For this review, take the finished solid that the model builds, in its own axes (mm). A direction names the side the tool comes from. Round coordinates to 2 decimals unless told otherwise and drop trailing zeros. Order: outer loops, then holes, each group sorted by start corner. A loop starts at its lowest first (then second) coordinate and runs counter-clockwise, first axis right, second up. Notation, with made-up numbers: M 1,62 L 12,62 A19 ccw 12,76 Z; hole C 73.5,-38.75 d3. An arc over 180 degrees is marked long. Use a Markdown table: item, result.
from build123d import *

# Parameters (mm, degrees)
SKETCH1_R           = 1.75
SKETCH1_W           = 3
SKETCH1_H           = 10
BOSS_EXTRUDE1_DEPTH = 3


with BuildPart() as part:
    # Sketch1 → Boss-Extrude1 (new body)
    with BuildSketch(Plane(origin=(0, 0, 0), x_dir=(1, 0, 0), z_dir=(0, 1, 0))):
        with BuildLine():
            Line((-32.051716829, -25), (-32.051716829, 2.5))
            ThreePointArc((-32.051716829, 2.5), (-34.980649017, 9.571067812), (-42.051716829, 12.5))
            Line((-42.051716829, 12.5), (-62.5, 12.5))
            ThreePointArc((-62.5, 12.5), (-64.267766953, 11.767766953), (-65, 10))
            Line((-65, 10), (-65, -10))
            ThreePointArc((-65, -10), (-64.267766953, -11.767766953), (-62.5, -12.5))
            Line((-62.5, -12.5), (-51.731989821, -12.5))
            ThreePointArc((-51.731989821, -12.5), (-47.304406502, -13.946364237), (-44.584529361, -17.727598413))
            Line((-44.584529361, -17.727598413), (-41.943571372, -26.034291608))
            ThreePointArc((-41.943571372, -26.034291608), (-36.531751789, -29.972890141), (-32.051716829, -25))
        make_face()
        with Locations(Location((-45, 0, 0), (0, 0, 270))):
            Circle(SKETCH1_R, mode=Mode.SUBTRACT)
        with Locations(Location((-37.051716829, -25, 0), (0, 0, 270))):
            Circle(SKETCH1_R, mode=Mode.SUBTRACT)
        with Locations((-59, 0)):
            Rectangle(SKETCH1_W, SKETCH1_H, mode=Mode.SUBTRACT)
    extrude(amount=BOSS_EXTRUDE1_DEPTH)


solid = part.part
Q1. Wall thickness on line 1 along X through (y, z) = (2.15, 0); line 2 along X through (y, z) = (1.75, 25); line 3 along Z through (x, y) = (-59, 0.7): over which ranges is each line inside the solid? List them lowest first. Write a range as [from, to].
Determined:
| item | result |
|---|---|
| line 1 | x = [-65, -60.5], [-57.5, -46.75], [-43.25, -32.05] |
| line 2 | x = [-42.27, -38.8], [-35.3, -32.05] |
| line 3 | z = [-12.5, -5], [5, 12.5] |
Q2. Add section C-C (x = -53.5). Write out the cut boundary in (y, z).
Determined:
| item | result |
|---|---|
| outline | M 0,-12.5 L 3,-12.5 L 3,12.5 L 0,12.5 Z |
Q3. Add section A-A (z = 0). Write out the cut boundary in (x, y).
Determined:
| item | result |
|---|---|
| outline | M -65,0 L -60.5,0 L -60.5,3 L -65,3 Z; M -57.5,0 L -46.75,0 L -46.75,3 L -57.5,3 Z; M -43.25,0 L -32.05,0 L -32.05,3 L -43.25,3 Z |
Q4. Add section B-B (y = 2.1). Write out the cut boundary in (x, z), then the cut area to 3 significant figures.
Determined:
| item | result |
|---|---|
| outline | M -65,-10 A2.5 ccw -62.5,-12.5 L -42.05,-12.5 A10 ccw -32.05,-2.5 L -32.05,25 A5 ccw -41.94,26.03 L -44.58,17.73 A7.5 cw -51.73,12.5 L -62.5,12.5 A2.5 ccw -65,10 Z; hole M -60.5,-5 L -57.5,-5 L -57.5,5 L -60.5,5 Z; hole C -45,0 d3.5; hole C -37.05,25 d3.5 |
| area | 948 mm^2 |
Q5. Draft analysis for pull direction X (two halves, no side actions). For faces 1 (the cylindrical face through (-64, 1, 12)), 2 (the flat face through (-45, 0, 4)), 3 (the cylindrical face through (-36.97, 1.48, 23.25)), 4 (the cylindrical face through (-37, 1, 30)), state which applies: pulls with the +X half, pulls with the -X half, needs draft (parallel to the pull), parting line crosses it, or undercut.
Determined:
| item | result |
|---|---|
| face 1 | pulls with the -X half |
| face 2 | needs draft |
| face 3 | undercut |
| face 4 | parting line crosses it |
Q6. Clearance check with flat-ended pins moving along their axes: pin 1 (1.5 mm diameter, centred on x = -59, y = 2, fed in from +Z); pin 2 (1 mm diameter, centred on x = -40.5, y = 0.5, fed in from -Z). State where each tip first meets the part, or that it passes through.
Determined:
| item | result |
|---|---|
| pin 1 | stops at z = 12.5 |
| pin 2 | stops at z = -12.44 |
Q7. Add section D-D (z = 13.5). Write out the cut boundary in (x, y).
Determined:
| item | result |
|---|---|
| outline | M -47.99,0 L -32.05,0 L -32.05,3 L -47.99,3 Z |
Q8. Machinability: for faces 5 (the flat face through (-32.052, 1, 11)), 6 (the flat face through (-57, 1, 12.5)), 7 (the flat face through (-60.5, 1, 0)), which of the approach directions +Z, -Z, +X, -X, +Y, -Y give a long, thin tool a straight path to every point of the face, cutting with its end or side? Answer none if there is none.
Determined:
| item | result |
|---|---|
| face 5 | +Z, -Z, +X, +Y, -Y |
| face 6 | +Z, -X, +Y, -Y |
| face 7 | +Y, -Y |
